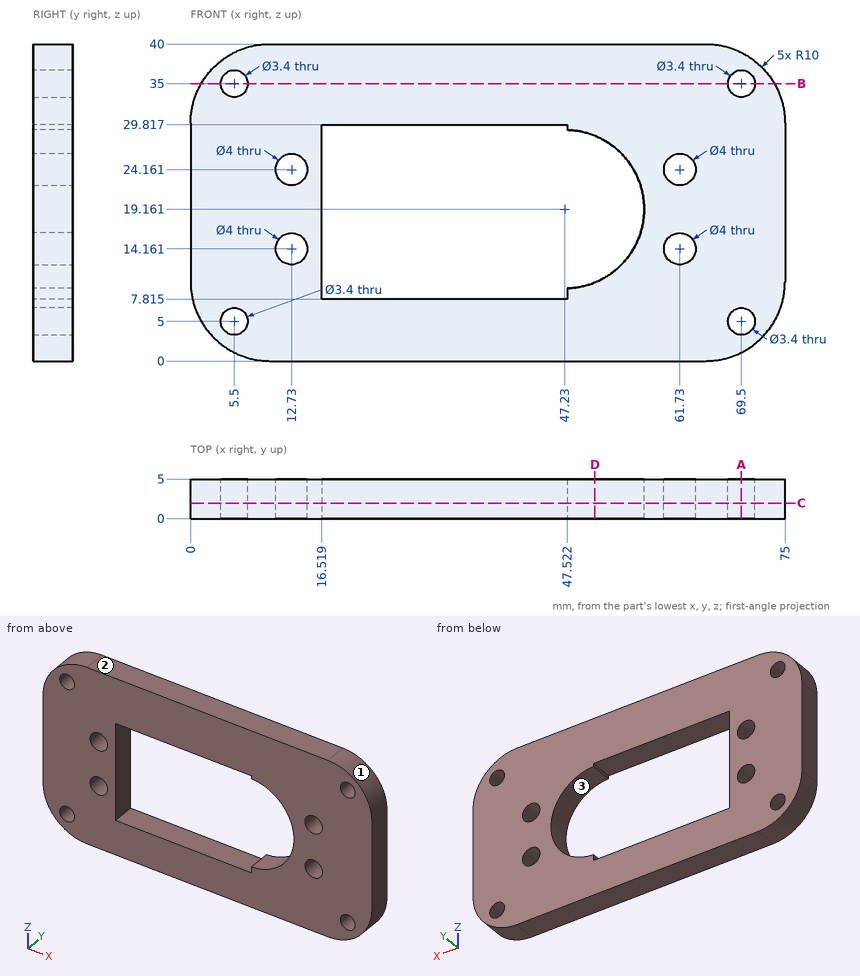
Check sheet for the drawn part. Datum: minimum x, y, z corner. Units: mm. Coordinates: 2 decimals unless noted, no trailing zeros. Loops run counter-clockwise (first coordinate to the right, second up) from the corner with the lowest first, then second, coordinate; pieces in that order, holes last. Notation, with made-up numbers: (4.5, -18.5) -> (28.5, -18.5) arc R10 cw to (28.5, -2.5) -> close; hole circle Ø1 at (-39.5, 73.5). An arc over 180 degrees is marked (long way). Answer in a Markdown table with one row per item.
1) Section check A-A (x = 69.5). Record the cut outline in (y, z), and give its area (3 significant figures).
The answers:
| item | result |
|---|---|
| outline | (0, 1.07) -> (5, 1.07) -> (5, 3.3) -> (0, 3.3) -> close; (0, 6.7) -> (5, 6.7) -> (5, 33.3) -> (0, 33.3) -> close; (0, 36.7) -> (5, 36.7) -> (5, 38.93) -> (0, 38.93) -> close |
| area | 155 mm2 |
2) Depth check by flat-ended pin: P1, Ø2.5, axis at x = 12.73, z = 14.16, coming from the -Y side; P2, Ø1.1, axis at y = 2.5, z = 8.5, coming from the -X side (1 decimal). Enter the tip coordinate at first touch or a pass-through.
The answers:
| item | result |
|---|---|
| P1 | passes through |
| P2 | stops at x = 0 |
3) Section check C-C (y = 1.95). Give the number of separate pieces and of enclosed holes in the cut face, and give its area (3 significant figures).
The answers:
| item | result |
|---|---|
| separate pieces | 1 |
| enclosed holes | 9 |
| area | 1,990 mm2 |
4) Scan lines: line 1 along X through (y, z) = (1.1, 5); line 2 along X through (y, z) = (2.85, 6) (1 decimal); line 3 along X through (y, z) = (1.3, 14.5). Record each from-to range of solid material in increasing order. Write a range as from..to.
The answers:
| item | result |
|---|---|
| line 1 | x = 1.34..3.8, 7.2..67.8, 71.2..73.66 |
| line 2 | x = 0.8..4.1, 6.9..68.1, 70.9..74.2 |
| line 3 | x = 0..10.76, 14.7..16.52, 56.08..59.76, 63.7..75 |
5) Section check D-D (x = 51). Record the cut outline in (y, z), and give its area (3 significant figures).
The answers:
| item | result |
|---|---|
| outline | (0, 0) -> (5, 0) -> (5, 9.9) -> (0, 9.9) -> close; (0, 28.42) -> (5, 28.42) -> (5, 40) -> (0, 40) -> close |
| area | 107 mm2 |
6) Draft check along X on the marked faces 1, 2 and 3. Enter one of: released by +X, released by -X, zero draft, split by the parting line, or undercut.
The answers:
| item | result |
|---|---|
| face 1 | released by +X |
| face 2 | zero draft |
| face 3 | undercut |
7) Section check B-B (z = 35). Record the cut outline in (x, y).
The answers:
| item | result |
|---|---|
| outline | (1.34, 0) -> (3.8, 0) -> (3.8, 5) -> (1.34, 5) -> close; (7.2, 0) -> (67.8, 0) -> (67.8, 5) -> (7.2, 5) -> close; (71.2, 0) -> (73.66, 0) -> (73.66, 5) -> (71.2, 5) -> close |
